Here's how the part is built. I have some questions about the finished solid (model axes, mm). Coordinates: 2 decimals unless noted, no trailing zeros. Write each loop counter-clockwise with the first axis right and the second up, starting at its lowest first coordinate (ties: lowest second). Pieces come first, ordered by that corner, then holes. Notation, with made-up numbers: (82, 66) -> (120, 66) arc R22 cw to (120, 90) -> close; hole circle Ø7 at (87, 43). An arc over 180 degrees is marked (long way). Use a Markdown table: item, result. Add a question column.
Item 1: Imagine slicing it at D-D, the plane x = -141.5. Write out the boundary of the cut face in (y, z).
Item 2: Imagine slicing it at A-A, the plane x = -128.5. Write out the boundary of the cut face in (y, z), and give its area (3 significant figures).
Item 3: Imagine slicing it at C-C, the plane y = -17.5. Write out the boundary of the cut face in (x, z).
Item 4: If I drill on line 1 along Y through (x, z) = (-129.5, 0.2); line 2 along Y through (x, z) = (-124, 0.7); line 3 along Y through (x, z) = (-129, 1.1), over which ranges is the centre line in solid material (lowest first)? Write a range as from..to.
Item 5: Will these pins go through, and if not, where does the flat tip stop? pin 1 Ø0.5 at (x, z) = (-139, 0.5) entering from -Y; pin 2 Ø0.5 at (x, z) = (-142.5, 1) entering from +Y; pin 3 Ø4 at (x, y) = (-124, -33.5) entering from -Z; pin 4 Ø0.5 at (y, z) = (-41, 0.5) entering from -X.
Item 6: Imagine slicing it at B-B, the plane z = 0.5. Write out the boundary of the cut face in (x, y), and give its area (3 significant figures).
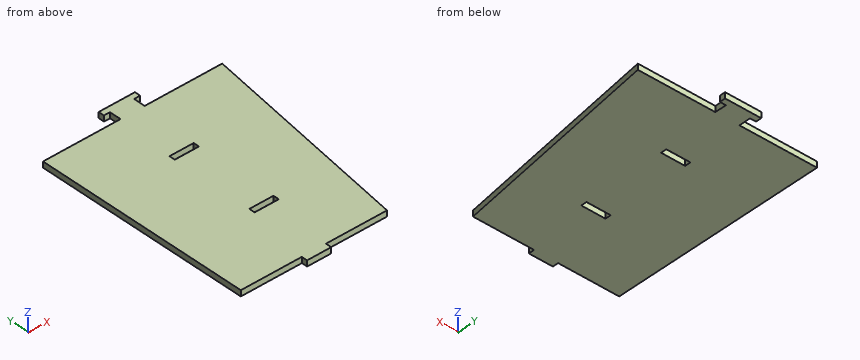
```python
from build123d import *

# Parameters (mm, degrees)
BOSS_EXTRUDE1_DEPTH = 1.524
SKETCH2_W           = 6.35
SKETCH2_H           = 1.524
CUT_EXTRUDE1_DEPTH  = 1.524


with BuildPart() as part:
    # Sketch1 → Boss-Extrude1 (new body)
    with BuildSketch(Plane.XY):
        Polygon((-102.477755775, -1.524), (-110.726395883, -58.314338926), (-126.787898899, -58.314338926), (-126.787898899, -59.838338926), (-133.137898899, -59.838338926), (-133.137898899, -58.314338926), (-149.199401915, -58.314338926), (-149.6392871, -1.524), (-129.233521437, -1.524), (-129.233521437, 1.524), (-130.821021437, 1.524), (-130.821021437, 3.048), (-121.296021437, 3.048), (-121.296021437, 1.524), (-122.883521437, 1.524), (-122.883521437, -1.524), align=None)
    extrude(amount=BOSS_EXTRUDE1_DEPTH)

    # Sketch2 → Cut-Extrude1 (cut)
    with BuildSketch(Plane.XY.offset(1.524)):
        with Locations((-127.078752717, -40.703047377)):
            Rectangle(SKETCH2_W, SKETCH2_H)
        with Locations((-127.078752717, -17.602011312)):
            Rectangle(SKETCH2_W, SKETCH2_H)
    extrude(amount=-CUT_EXTRUDE1_DEPTH, mode=Mode.SUBTRACT)


solid = part.part
```
Ans:
| question | item | result |
|---|---|---|
| 1 | outline | (-58.31, 0) -> (-1.52, 0) -> (-1.52, 1.52) -> (-58.31, 1.52) -> close |
| 2 | outline | (-59.84, 0) -> (-41.47, 0) -> (-41.47, 1.52) -> (-59.84, 1.52) -> close; (-39.94, 0) -> (-18.36, 0) -> (-18.36, 1.52) -> (-39.94, 1.52) -> close; (-16.84, 0) -> (3.05, 0) -> (3.05, 1.52) -> (-16.84, 1.52) -> close |
| 2 | area | 91.2 mm^2 |
| 3 | outline | (-149.52, 0) -> (-130.25, 0) -> (-130.25, 1.52) -> (-149.52, 1.52) -> close; (-123.9, 0) -> (-104.8, 0) -> (-104.8, 1.52) -> (-123.9, 1.52) -> close |
| 4 | line 1 | y = -59.84..-41.47, -39.94..-18.36, -16.84..-1.52, 1.52..3.05 |
| 4 | line 2 | y = -58.31..-41.47, -39.94..-18.36, -16.84..3.05 |
| 4 | line 3 | y = -59.84..-41.47, -39.94..-18.36, -16.84..3.05 |
| 5 | pin 1 | stops at y = -58.31 |
| 5 | pin 2 | stops at y = -1.52 |
| 5 | pin 3 | stops at z = 0 |
| 5 | pin 4 | stops at x = -149.34 |
| 6 | outline | (-149.64, -1.52) -> (-149.2, -58.31) -> (-133.14, -58.31) -> (-133.14, -59.84) -> (-126.79, -59.84) -> (-126.79, -58.31) -> (-110.73, -58.31) -> (-102.48, -1.52) -> (-122.88, -1.52) -> (-122.88, 1.52) -> (-121.3, 1.52) -> (-121.3, 3.05) -> (-130.82, 3.05) -> (-130.82, 1.52) -> (-129.23, 1.52) -> (-129.23, -1.52) -> close; hole (-130.25, -41.47) -> (-123.9, -41.47) -> (-123.9, -39.94) -> (-130.25, -39.94) -> close; hole (-130.25, -18.36) -> (-123.9, -18.36) -> (-123.9, -16.84) -> (-130.25, -16.84) -> close |
| 6 | area | 2,460 mm^2 |
